Source: CAD feature listing. Evaluate the final solid. Frame: model axes, mm. A direction names the side the tool comes from. Coordinates: 2 decimals unless noted, no trailing zeros. Order: outer loops, then holes, each group sorted by start corner. A loop starts at its lowest first (then second) coordinate and runs counter-clockwise, first axis right, second up.
```python
from build123d import *

# Parameters (mm, degrees)
F0_R     = 1.5
F1_DEPTH = 3
F2_DEPTH = 1.5


with BuildPart() as f1:
    # F0 (on Front) → F1 (new body)
    with BuildSketch(Plane.XZ):
        with BuildLine():
            Line((-6, -9.2712371871), (-6, -6.2712371871))
            Line((-6, -6.2712371871), (0, -6.2712371871))
            Line((0, -6.2712371871), (6, -6.2712371871))
            Line((6, -6.2712371871), (6, 0))
            Line((6, 0), (6, 12.7287628129))
            ThreePointArc((6, 12.7287628129), (0, 18.7287628129), (-6, 12.7287628129))
            Line((-6, 12.7287628129), (-7.5, 5.7287628129))
            Line((-7.5, 5.7287628129), (-7.5, -6.2712371871))
            Line((-7.5, -6.2712371871), (-7.5, -12.1941817924))
            Line((-7.5, -12.1941817924), (-6, -12.1941817924))
            Line((-6, -12.1941817924), (-6, -12.2712371871))
            Line((-6, -12.2712371871), (0, -12.2712371871))
            Line((0, -12.2712371871), (6, -12.2712371871))
            Line((6, -12.2712371871), (6, -9.2712371871))
            Line((6, -9.2712371871), (0, -9.2712371871))
            Line((0, -9.2712371871), (-6, -9.2712371871))
        make_face()
        with Locations((0, 12.7287628129)):
            Circle(F0_R, mode=Mode.SUBTRACT)
    extrude(amount=F1_DEPTH)

    # F0 (on Front) → F2 (join)
    with BuildSketch(Plane.XZ):
        Polygon((0, -6.2712371871), (-6, -6.2712371871), (-6, -9.2712371871), (0, -9.2712371871), (6, -9.2712371871), (6, -6.2712371871), align=None)
    extrude(amount=F2_DEPTH)


solid = f1.part
```
1. Section query B-B on y = -2.3. Return loops of the section in (x, z).
Findings:
outline: (-7.5, -12.19) - (-6, -12.19) - (-6, -12.27) - (6, -12.27) - (6, -9.27) - (-6, -9.27) - (-6, -6.27) - (6, -6.27) - (6, 12.73) arc R6 ccw to (-6, 12.73) - (-7.5, 5.73) - close; hole circle Ø3 at (0, 12.73)
2. Section query D-D on x = 3.75. Return loops of the section in (y, z).
Findings:
outline: (-3, -12.27) - (0, -12.27) - (0, 17.41) - (-3, 17.41) - (-3, -6.27) - (-1.5, -6.27) - (-1.5, -9.27) - (-3, -9.27) - close
3. Section query A-A on x = 0. Return loops of the section in (y, z), plus the area to 3 significant figures.
Findings:
outline: (-3, -12.27) - (0, -12.27) - (0, 11.23) - (-3, 11.23) - (-3, -6.27) - (-1.5, -6.27) - (-1.5, -9.27) - (-3, -9.27) - close; (-3, 14.23) - (0, 14.23) - (0, 18.73) - (-3, 18.73) - close
area: 79.5 mm2
4. Access query for faces 5 (the face through (0, -1.5, -8)), 6 (the face through (6, -1, 0)), 7 (the face through (-7, -1, -12.194)). Directions: +Z, -Z, +X, -X, +Y, -Y. A direction counts if a zero-diameter tool reaches every point of the face in a straight line with its end or side. Return the directions, or none.
Findings:
face 5: +X, -Y
face 6: +Z, -Z, +X, +Y, -Y
face 7: -Z, -X, +Y, -Y
5. Draft query along X for faces 1 (the face through (0.132, -1.479, 18.727)), 2 (the face through (-1, 0, 3)), 3 (the face through (-0.325, -1.479, 11.264)), 4 (the face through (-6.74, -1.48, 9.28)). Return one class per face: released by +X, released by -X, zero draft, split by the parting line, or undercut.
Findings:
face 1: split by the parting line
face 2: zero draft
face 3: undercut
face 4: released by -X
6. Ray query, line 1 (Z direction, x = 0, y = -1.6); line 2 (Z direction, x = 0, y = -0.7); line 3 (Y direction, x = 4.25, z = -9). Return the intervals inside material, ascending.
Findings:
line 1: z = -12.27 to -9.27, -6.27 to 11.23, 14.23 to 18.73
line 2: z = -12.27 to 11.23, 14.23 to 18.73
line 3: y = -1.5 to 0
7. Pin query (flat end, axial travel): P1, Ø2.5, axis at x = -0.5, z = -7, coming from the -Y side. Return the tip coordinate at first contact, or that it passes through.
Findings:
P1: stops at y = -3
8. Section query C-C on z = -7. Return loops of the section in (x, y), plus the area to 3 significant figures.
Findings:
outline: (-7.5, -3) - (-6, -3) - (-6, -1.5) - (6, -1.5) - (6, 0) - (-7.5, 0) - close
area: 22.5 mm2
